from build123d import *

# Parameters (mm, degrees)
SKETCH_1_W            = 533
SKETCH_1_H            = 398
EXTRUDE_237_DEPTH     = 60
SKETCH_2_R            = 86.5
CUT_EXTRUDE_597_DEPTH = 20
SKETCH_3_R            = 53
CUT_EXTRUDE_101_DEPTH = 15
SKETCH_6_R            = 43
CUT_EXTRUDE_5_DEPTH   = 14
SKETCH_7_R            = 30
CUT_EXTRUDE_6_DEPTH   = 12


with BuildPart() as part:
    # Эскиз1 → Extrude 237 (new body)
    with BuildSketch(Plane(origin=(0, 0, 0), x_dir=(1, 0, 0), z_dir=(0, 1, 0))):
        with Locations((266.5, 199)):
            Rectangle(SKETCH_1_W, SKETCH_1_H)
    extrude(amount=-EXTRUDE_237_DEPTH)

    # Эскиз2 → Р597 (cut)
    with BuildSketch(Plane(origin=(0, 0, 0), x_dir=(1, 0, 0), z_dir=(0, 1, 0))):
        with Locations(Location((429.166666667, 103.833333333, 0), (0, 0, 270))):
            Circle(SKETCH_2_R)
        with Locations(Location((238.833333333, 103.833333333, 0), (0, 0, 270))):
            Circle(SKETCH_2_R)
        with Locations(Location((238.833333333, 294.166666667, 0), (0, 0, 270))):
            Circle(SKETCH_2_R)
        with Locations(Location((429.166666667, 294.166666667, 0), (0, 0, 270))):
            Circle(SKETCH_2_R)
    extrude(amount=-CUT_EXTRUDE_597_DEPTH, mode=Mode.SUBTRACT)

    # Эскиз3 → КМЕ-101 (cut)
    with BuildSketch(Plane(origin=(0, 0, 0), x_dir=(1, 0, 0), z_dir=(0, 1, 0))):
        with Locations(Location((81, 283, 0), (0, 0, 270))):
            Circle(SKETCH_3_R)
        with Locations(Location((81, 115, 0), (0, 0, 270))):
            Circle(SKETCH_3_R)
    extrude(amount=-CUT_EXTRUDE_101_DEPTH, mode=Mode.SUBTRACT)

    # Эскиз6 → Вырез-Вытянуть5 (cut)
    with BuildSketch(Plane(origin=(0, -15, 0), x_dir=(1, 0, 0), z_dir=(0, 1, 0))):
        with Locations(Location((81, 283, 0), (0, 0, 270))):
            Circle(SKETCH_6_R)
        with Locations(Location((81, 115, 0), (0, 0, 270))):
            Circle(SKETCH_6_R)
    extrude(amount=-CUT_EXTRUDE_5_DEPTH, mode=Mode.SUBTRACT)

    # Эскиз7 → Вырез-Вытянуть6 (cut)
    with BuildSketch(Plane(origin=(0, -29, 0), x_dir=(1, 0, 0), z_dir=(0, 1, 0))):
        with Locations(Location((81, 283, 0), (0, 0, 270))):
            Circle(SKETCH_7_R)
        with Locations(Location((81, 115, 0), (0, 0, 270))):
            Circle(SKETCH_7_R)
    extrude(amount=-CUT_EXTRUDE_6_DEPTH, mode=Mode.SUBTRACT)


solid = part.part
Read the model definition and answer for the solid it produces. Units are mm, in the model's axes. A direction names the side the tool comes from. Give positions to 0.01 mm unless a question says otherwise; leave off trailing zeros. Write each loop counter-clockwise with the first axis right and the second up, starting at its lowest first coordinate (ties: lowest second). Pieces come first, ordered by that corner, then holes. Notation, with made-up numbers: (79, 16.25) - (92, 16.25) arc R28 cw to (92, 52.25) - close; hole circle Ø7 at (33.5, 25.25). An arc over 180 degrees is marked (long way). Use CSV: the item, a comma, the result in double quotes. Start each with the question number.
Item 1: The part is cut by section C-C, the plane x = 392.5. Give the vertices of the cut face in (y, z).
Item 2: The part is cut by section B-B, the plane z = -97. Give the vertices of the cut face in (x, y).
Item 3: The mould has two halves that part along X. Classify faces 3 (the flat face through (533, -30, -196)), 4 (the flat face through (81, -41, -283)), 5 (the flat face through (204, 0, -202)), 6 (the cylindrical face through (297.29, -9.86, -167.59)): pulls with the +X half, pulls with the -X half, needs draft (parallel to the pull), parting line crosses it, or undercut.
Item 4: The part is cut by section A-A, the plane x = 81. Give the vertices of the cut face in (y, z).
Item 5: Consider line 1 (X direction, y = -32, z = -115); line 2 (Z direction, x = 283, y = -15.5); line 3 (Z direction, x = 501, y = -14.5). Determine where each line is inside the solid, lowest interval first.
Item 6: The part is cut by section D-D, the plane z = -342. Give the vertices of the cut face in (x, y).
Item 7: Flat-ended cylindrical pins translate along their axes: P1, Ø12, axis at x = 230.5, z = -270.5, coming from the +Y side; P2, Ø2, axis at x = 289.5, z = -207.5, coming from the +Y side. Find the tip coordinate at first contact, or state that the pin passes through.
Item 8: For faces 1 (the cylindrical face through (264.816, -9.86, -211.661)), 2 (the flat face through (263, -60, -202)), determine the directions among +Z, -Z, +X, -X, +Y, -Y from which every point of the face is accessible in a straight line to the end or side of a thin tool.
Taken from the geometry:
1,outline,"(-60, -398) - (0, -398) - (0, -372.51) - (-20, -372.51) - (-20, -215.82) - (0, -215.82) - (0, -182.18) - (-20, -182.18) - (-20, -25.49) - (0, -25.49) - (0, 0) - (-60, 0) - close"
2,outline,"(0, -60) - (533, -60) - (533, 0) - (515.4, 0) - (515.4, -20) - (342.94, -20) - (342.94, 0) - (325.06, 0) - (325.06, -20) - (152.6, -20) - (152.6, 0) - (130.85, 0) - (130.85, -15) - (120.05, -15) - (120.05, -29) - (105, -29) - (105, -41) - (57, -41) - (57, -29) - (41.95, -29) - (41.95, -15) - (31.15, -15) - (31.15, 0) - (0, 0) - close"
3,face 3,"pulls with the +X half"
3,face 4,"undercut"
3,face 5,"needs draft"
3,face 6,"undercut"
4,outline,"(-60, -398) - (0, -398) - (0, -336) - (-15, -336) - (-15, -326) - (-29, -326) - (-29, -313) - (-41, -313) - (-41, -253) - (-29, -253) - (-29, -240) - (-15, -240) - (-15, -230) - (0, -230) - (0, -168) - (-15, -168) - (-15, -158) - (-29, -158) - (-29, -145) - (-41, -145) - (-41, -85) - (-29, -85) - (-29, -72) - (-15, -72) - (-15, -62) - (0, -62) - (0, 0) - (-60, 0) - close"
5,line 1,"0 to 51, 111 to 533"
5,line 2,"-398 to -368.54, -219.79 to -178.21, -29.46 to 0"
5,line 3,"-398 to -342.36, -245.98 to -152.02, -55.64 to 0"
6,outline,"(0, -60) - (533, -60) - (533, 0) - (501.24, 0) - (501.24, -20) - (357.1, -20) - (357.1, 0) - (310.9, 0) - (310.9, -20) - (166.76, -20) - (166.76, 0) - (0, 0) - close"
7,P1,"y = -20"
7,P2,"y = 0"
8,face 1,"+Y"
8,face 2,"+Z, -Z, +X, -X, -Y"
